Part model, mm, in its own coordinate system. A direction names the side the tool comes from. Coordinates: 2 decimals unless noted, no trailing zeros. Loops run counter-clockwise (first coordinate to the right, second up) from the corner with the lowest first, then second, coordinate; pieces in that order, holes last. Notation, with made-up numbers: M -26.75,19.25 L 2.25,19.25 A10 cw 2.25,31.25 Z; hole C -14,82.25 d9. An arc over 180 degrees is marked long. Answer as a JSON object with one key per item and string values. Group by question number.
1. Saw through at B-B on x = -6.5. Write the cut outline in (y, z).
2. Drill centre lines: L1, parallel to Z at x = -0.5, y = -13; L2, parallel to Y at x = -9, z = -16; L3, parallel to Z at x = -4, y = -9.5. Where is each one in solid material? Low to high.
3. Saw through at D-D on x = -17. Write the cut outline in (y, z).
4. Drop flat-ended pins along their axis: pin 1 Ø1 at (y, z) = (-14.5, 5.5) entering from -X; pin 2 Ø2 at (x, y) = (-7, -41.5) entering from -Z; pin 3 Ø2 at (y, z) = (-26.5, -5.5) entering from +X. Give the stop position or say it passes through.
5. 3-axis set-ups, long thin cutter, end or side, ignore diameter. For faces 1 (the face through (-11.651, -26.798, -8.934)), 2 (the face through (12.5, 1.1, -12.9)): which of +Z, -Z, +X, -X, +Y, -Y reach the whole face in a straight line?
6. Mould opens along Z. For faces 3 (the face through (-12.5, 1.1, 12.9)), 4 (the face through (11.817, -26.431, -4.9)), 5 (the face through (-11, 0, 10)), 6 (the face through (-12.9, 1.1, -12.5)) say: released by +Z, released by -Z, zero draft, split by the parting line, or undercut.
7. Saw through at C-C on y = -23. Write the cut outline in (x, z), then the cut area to 3 significant figures.
8. Saw through at A-A on z = -4.5. Write the cut outline in (x, y).
from build123d import *

# Parameters (mm, degrees)
F2_DEPTH = 2.286
F1_R     = 14.68178
F3_DEPTH = 54.356
F4_R     = 12.792611
F5_DEPTH = 76.2


with BuildPart() as f2:
    # F0 (on Front) → F2 (new body)
    with BuildSketch(Plane.XZ):
        Polygon((0, 25.4), (-25.4, 0), (0, -25.4), (25.4, 0), align=None)
    extrude(amount=-F2_DEPTH)

    # F1 (on Front) → F3 (join)
    with BuildSketch(Plane.XZ):
        Circle(F1_R)
    extrude(amount=F3_DEPTH)

    # F4 (on face) → F5 (cut)
    with BuildSketch(Plane.XZ.offset(54.356)):
        Circle(F4_R)
    extrude(amount=-F5_DEPTH, mode=Mode.SUBTRACT)


solid = f2.part
Outcome:
{
 "1": {"outline": "M -54.36,-13.16 L 0,-13.16 L 0,-18.9 L 2.29,-18.9 L 2.29,-11.02 L -54.36,-11.02 Z; M -54.36,11.02 L 2.29,11.02 L 2.29,18.9 L 0,18.9 L 0,13.16 L -54.36,13.16 Z"},
 "2": {"L1": "z = -14.67 to -12.78, 12.78 to 14.67", "L2": "y = 0 to 2.29", "L3": "z = -14.13 to -12.15, 12.15 to 14.13"},
 "3": {"outline": "M 0,-8.4 L 2.29,-8.4 L 2.29,8.4 L 0,8.4 Z"},
 "4": {"pin 1": "stops at x = -13.8", "pin 2": "stops at z = -13.4", "pin 3": "stops at x = 13.98"},
 "5": {"face 1": "-Y", "face 2": "-Z, +X, +Y, -Y"},
 "6": {"face 3": "released by +Z", "face 4": "undercut", "face 5": "zero draft", "face 6": "released by -Z"},
 "7": {"outline": "C 0,0 d29.36; hole C 0,0 d25.59", "area": "163 mm²"},
 "8": {"outline": "M -20.9,0 L -13.98,0 L -13.98,-54.36 L -11.98,-54.36 L -11.98,2.29 L -20.9,2.29 Z; M 11.98,-54.36 L 13.98,-54.36 L 13.98,0 L 20.9,0 L 20.9,2.29 L 11.98,2.29 Z"}
}
